```python
from build123d import *

# Parameters (mm, degrees)
BOSS_EXTRUDE1_DEPTH     = 250
SKETCH3_R               = 78
BOSS_EXTRUDE2_DEPTH     = 5
SKETCH4_W               = 20
SKETCH4_H               = 50
BOSS_EXTRUDE3_DEPTH     = 8
SKETCH5_R               = 56
BOSS_EXTRUDE4_DEPTH     = 5
SKETCH6_W               = 140.323042475
SKETCH6_H               = 120
BOSS_EXTRUDE5_DEPTH     = 8
CUT_EXTRUDE1_DEPTH      = 619.973343529
CUT_EXTRUDE1_DEPTH_BACK = 619.973343529
CUT_EXTRUDE2_DEPTH      = 619.973343529
CUT_EXTRUDE2_DEPTH_BACK = 619.973343529


with BuildPart() as part:
    # Sketch2 → Boss-Extrude1 (new body)
    with BuildSketch(Plane.XY):
        with BuildLine():
            Line((0, 0), (0, -258))
            Line((0, -258), (500, -258))
            Line((500, -258), (500, -48))
            Line((500, -48), (405.149093968, -79.675))
            ThreePointArc((405.149093968, -79.675), (279.704330156, -61.001338916), (220.815553876, 51.325))
            Line((220.815553876, 51.325), (140.816338804, 51.679383953))
            Line((140.816338804, 51.679383953), (0, 0))
        make_face()
    extrude(amount=-BOSS_EXTRUDE1_DEPTH)

    # Sketch3 → Boss-Extrude2 (add)
    with BuildSketch(Plane.XY):
        with Locations(Location((147.365575326, -47.984465758, 0), (0, 0, 180))):
            Circle(SKETCH3_R)
    extrude(amount=BOSS_EXTRUDE2_DEPTH)

    # Sketch4 → Boss-Extrude3 (add)
    with BuildSketch(Plane.XY):
        with Locations((33.562653109, -47.515690105)):
            Rectangle(SKETCH4_W, SKETCH4_H)
    extrude(amount=BOSS_EXTRUDE3_DEPTH)

    # Sketch5 → Boss-Extrude4 (add)
    with BuildSketch(Plane(origin=(0, 0, -250), x_dir=(-1, 0, 0), z_dir=(0, 0, -1))):
        with Locations((-147.365575326, -47.984465758)):
            Circle(SKETCH5_R)
    extrude(amount=BOSS_EXTRUDE4_DEPTH)

    # Sketch6 → Boss-Extrude5 (add)
    with BuildSketch(Plane(origin=(0, 0, -250), x_dir=(-1, 0, 0), z_dir=(0, 0, -1))):
        with Locations((-147.365575326, -182.265748938)):
            Rectangle(SKETCH6_W, SKETCH6_H)
    extrude(amount=BOSS_EXTRUDE5_DEPTH)

    # Sketch8 → Cut-Extrude1 (cut, two sides: drawn at the far end of the back side and taken through both)
    with BuildSketch(Plane(origin=(0, 0, -250), x_dir=(-1, 0, 0), z_dir=(0, 0, -1)).offset(-CUT_EXTRUDE1_DEPTH_BACK)):
        Polygon((-500, -78.40253223), (-500, -258), (-457.637340455, -99.900402235), (-448.352137529, -65.247553157), (-500, -48), align=None)
    extrude(amount=CUT_EXTRUDE1_DEPTH + CUT_EXTRUDE1_DEPTH_BACK, mode=Mode.SUBTRACT)

    # Sketch9 → Cut-Extrude2 (cut, two sides: drawn at the far end of the back side and taken through both)
    with BuildSketch(Plane(origin=(0, 0, -250), x_dir=(-1, 0, 0), z_dir=(0, 0, -1)).offset(-CUT_EXTRUDE2_DEPTH_BACK)):
        Polygon((-65.451377524, -78.173818182), (0, -258), (0, -19.248703784), (0, 0), (-108.38155171, 39.77586601), align=None)
    extrude(amount=CUT_EXTRUDE2_DEPTH + CUT_EXTRUDE2_DEPTH_BACK, mode=Mode.SUBTRACT)


solid = part.part
```
Here's how the part is built. I have some questions about the finished solid (model axes, mm). A direction names the side the tool comes from. Coordinates: 2 decimals unless noted, no trailing zeros. Order: outer loops, then holes, each group sorted by start corner. A loop starts at its lowest first (then second) coordinate and runs counter-clockwise, first axis right, second up. Notation, with made-up numbers: M 10.5,6.5 L 59.5,6.5 A12 cw 59.5,20.5 Z; hole C 87.25,74.5 d8. An arc over 180 degrees is marked long. Answer as a JSON object with one key per item and string values. Group by question number.
(1) Suppose I cut it at D-D, the plane y = -113. Please give me the cut outline in (x, z), then the cut area to 3 significant figures.
(2) I need wall thicknesses on probe 1 along Y at (x, z) = (162, -163); probe 2 along Z at (x, y) = (100, -153); probe 3 along Z at (x, y) = (364.5, -147). Which ranges of each line are inside material? Lowest first, please.
(3) Suppose I cut it at B-B, the plane y = -71.5. Please give me the cut outline in (x, z), then the cut area to 3 significant figures.
(4) For pin 1 (5 mm diameter, centred on y = -123, z = -219, fed in from -X); pin 2 (1 mm diameter, centred on x = 261.5, y = -167, fed in from +Z); pin 3 (8 mm diameter, centred on y = -171, z = -128, fed in from +X), each with a flat end and sliding along its axis, tell me the tip position at first contact or that it passes through.
(5) If we mould it in two halves opening along Y, with no side actions, what happens to faces 1 (the face through (154.66, 7.54, -252.46)), 2 (the face through (149, -49, 5)), 3 (the face through (281.213, -62.059, -123.25))? For each: released by +Y, released by -Y, zero draft, split by the parting line, or undercut.
(6) Suppose I cut it at A-A, the plane z = -12.5. Please give me the cut outline in (x, y) (3 decimals), then the cut area to 3 significant figures.
(7) Which directions (+Z, -Z, +X, -X, +Y, -Y) give clear straight access to the entire face, cutting with the end or side of a thin tool? Please do faces 4 (the face through (148, -47, -255)), 5 (the face through (427.05, -72.36, -123.25)), 6 (the face through (219.644, -77.307, 2.465)).
(8) Suppose I cut it at C-C, the plane x = 156. Please give me the cut outline in (y, z).
Values found:
{
 "1": {"outline": "M 52.78,-250 L 461.15,-250 L 461.15,0 L 190.46,0 L 190.46,5 L 104.27,5 L 104.27,0 L 52.78,0 Z", "area": "103,000 mm^2"},
 "2": {"probe 1": "y = -258 to 51.59", "probe 2": "z = -258 to 0", "probe 3": "z = -250 to 0"},
 "3": {"outline": "M 67.88,-250 L 96.54,-250 L 96.54,-255 L 198.19,-255 L 198.19,-250 L 297,-250 L 297,0 L 221.74,0 L 221.74,5 L 72.99,5 L 72.99,0 L 67.88,0 Z; M 429.63,-250 L 450.03,-250 L 450.03,0 L 429.63,0 Z", "area": "63,600 mm^2"},
 "4": {"pin 1": "stops at x = 48.23", "pin 2": "stops at z = 0", "pin 3": "stops at x = 477.76"},
 "5": {"face 1": "undercut", "face 2": "zero draft", "face 3": "released by +Y"},
 "6": {"outline": "M 0,-258 L 500,-258 L 448.352,-65.248 L 405.149,-79.675 A140 cw 220.816,51.325 L 140.816,51.679 L 108.382,39.776 Z", "area": "99,600 mm^2"},
 "7": {"face 4": "-Z, +X, -X, +Y", "face 5": "+Z, -Z, +Y", "face 6": "+Z"},
 "8": {"outline": "M -258,-250 L -242.27,-250 L -242.27,-258 L -122.27,-258 L -122.27,-250 L -103.31,-250 L -103.31,-255 L 7.35,-255 L 7.35,-250 L 51.61,-250 L 51.61,0 L 29.54,0 L 29.54,5 L -125.51,5 L -125.51,0 L -258,0 Z"}
}
